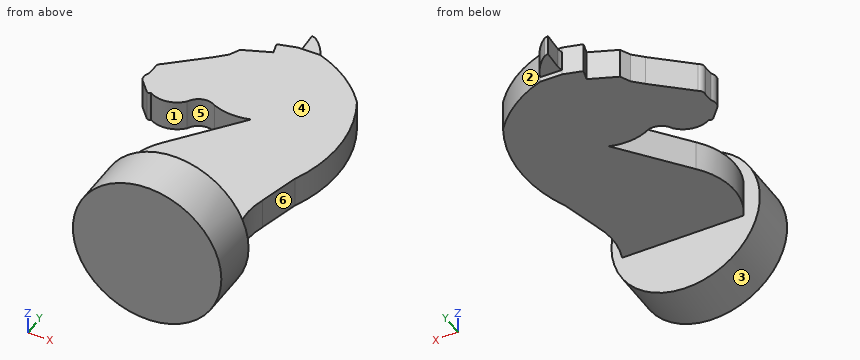
Autodesk Fusion 360 part; units mm, degrees
sketch "Base" plane through (0, 0, 0) normal (0, 0, 1) x (1, 0, 0)
  line L0 (1.35, -11.2) -> (8.7, -11.2)
  line L1 (8.7, -11.2) -> (8.7, -16.1)
  line L2 (8.7, -16.1) -> (1.35, -16.1)
  line L3 (1.35, -16.1) -> (1.35, -11.2)
  line L4 (1.35, -11.2) -> (1.35, -16.5) construction
revolve "Revolve1" add sketch "Base" angle 360 about axis through (1.35, -11.2, 0) along (0, -1, 0)
sketch "Sketch5" plane through (0, 0, 0) normal (0, 0, 1) x (1, 0, 0)
  line L0 (-3.8612, -3.6216) -> (1.2602, 2.7884)
  arc A0 (-2.4491, 2.9542) -> (-4.7968, 2.2709) centre (-3.3362, 1.6273) ccw
  arc A1 (-8.56, 1.8217) -> (-8.1023, 1.7795) centre (-8.3154, 1.9715) ccw
  arc A2 (-8.1023, 1.7795) -> (-4.7968, 2.2709) centre (-6.7484, 4.0355) ccw
  line L1 (-8.4888, 1.7431) -> (-9.6537, 3.0304)
  arc A3 (-9.5649, 4.0683) -> (-9.6537, 3.0304) centre (-8.6269, 3.4652) ccw
  line L2 (-9.5649, 4.0683) -> (-9.5, 4.9)
  arc A4 (-8.7221, 5.7752) -> (-9.5, 4.9) centre (-8.9, 5.15) ccw
  line L3 (-9.1971, 5.7281) -> (-5.657, 8.7735)
  arc A5 (-2.8723, 3.1545) -> (1.2602, 2.7884) centre (-0.3699, 7.8942) ccw
  line L4 (-3.8561, -11.9399) -> (7.9881, -11.9399)
  arc A6 (-3.8612, -3.6216) -> (-3.8561, -11.9399) centre (1.0426, -7.7778) ccw
  line L5 (-5.657, 8.7735) -> (-4.7, 9.7)
  line L6 (-4.7, 9.7) -> (-4.2, 10.7)
  line L7 (-4.2, 10.7) -> (-1.5, 11.8)
  line L8 (-1.5, 11.8) -> (-1.8, 12.9)
  line L9 (-1.8, 12.9) -> (0.0589, 13.407)
  line L10 (0.1583, 14.0219) -> (0.05, 16.1)
  arc A7 (0.0589, 13.407) -> (0.1571, 14.0443) centre (-1.3706, 13.9535) ccw
  arc A8 (2.2064, 13.4396) -> (0.05, 16.1) centre (-2.8988, 11.5057) ccw
  arc A9 (8.1474, 9.2996) -> (2.2064, 13.4396) centre (-1.7746, 1.394) ccw
  line L11 (8.5157, -2.5354) -> (7.2902, -7.2588)
  arc A10 (0.4921, 15.7841) -> (0.0594, 15.92) centre (-3.7578, 3.0059) ccw
  arc A11 (8.5157, -2.5354) -> (8.1474, 9.2996) centre (-3.7578, 3.0059) ccw
  arc A12 (7.4885, -6.4944) -> (7.9881, -11.9399) centre (14.1451, -8.6294) ccw
  line L12 (2.2064, 13.4396) -> (0.0589, 13.407)
extrude "Extrude1" add sketch "Sketch5" along normal mid plane 3 contours L0 A0 A1 A2 L1 A3 L2 A4 L3 A5 L4 A6 L5 L6 L7 L8 L9 A9 L11 A11 A12 L12
extrude "Extrude2" add sketch "Sketch5" along normal mid plane 2 contours L10 A7 A8 A10 L12
Input: part model. Units: mm. Frame: model coordinates. Face numbers are marked on the shaded views. A direction names the side the tool comes from. Round coordinates to 2 decimals unless told otherwise and drop trailing zeros. Loops run counter-clockwise (first coordinate to the right, second up) from the corner with the lowest first, then second, coordinate; pieces in that order, holes last. Notation, with made-up numbers: (81.25, 40.5) -> (98.25, 40.5) arc R21 cw to (98.25, 72.5) -> close; hole circle Ø6 at (4.25, 80.25). An arc over 180 degrees is marked (long way). Answer as a JSON object with one key per item and string values. Group by question number.
1) Draft query along X for the marked faces 1, 2 and 3. Return one class per face: +X half, -X half, draft (parallel to the pull), parting line (faces both ways), or undercut.
2) Pin query (flat end, axial travel): pin 1 (4 mm diameter, centred on y = -5, z = -1, fed in from +X); pin 2 (3 mm diameter, centred on x = -2, z = 1, fed in from +Y); pin 3 (1.1 mm diameter, centred on x = 0.5, y = 15, fed in from +Z). Return the tip coordinate at first contact, or that it passes through.
3) Section query A-A on x = -3.5. Output: boundary loops of the cut face in (y, z) (3 decimals), plus the area to 3 significant figures.
4) Reachability of the marked faces 4, 5 and 6 from +Z, -Z, +X, -X, +Y, -Y: full face, straight path, thin tool, end or side. Return the list, or none.
5) Section query D-D on y = -0.5. Output: boundary loops of the cut face in (x, z).
6) Section query C-C on x = 5.75. Output: boundary loops of the cut face in (y, z), plus the area to 3 significant figures.
7) Ray query, L1, parallel to Z at x = 0.25, y = 8; L2, parallel to Y at x = 1.5, z = 5; L3, parallel to Y at x = -2.75, z = 1. Return the intervals inside material, ascending.
Reply:
{
 "1": {"face 1": "undercut", "face 2": "+X half", "face 3": "parting line"},
 "2": {"pin 1": "stops at x = 8.4", "pin 2": "stops at y = 13.25", "pin 3": "stops at z = 1"},
 "3": {"outline": "(-16.1, -5.523) -> (-11.2, -5.523) -> (-11.2, -1.5) -> (-3.17, -1.5) -> (-3.17, 1.5) -> (-11.2, 1.5) -> (-11.2, 5.523) -> (-16.1, 5.523) -> close; (3.215, -1.5) -> (10.985, -1.5) -> (10.985, 1.5) -> (3.215, 1.5) -> close", "area": "102 mm2"},
 "4": {"face 4": "+Z, +X, -X, +Y", "face 5": "+Z, -Z", "face 6": "+Z, -Z, +X"},
 "5": {"outline": "(-1.37, -1.5) -> (9.24, -1.5) -> (9.24, 1.5) -> (-1.37, 1.5) -> close"},
 "6": {"outline": "(-16.1, -5.89) -> (-11.2, -5.89) -> (-11.2, -1.5) -> (11.61, -1.5) -> (11.61, 1.5) -> (-11.2, 1.5) -> (-11.2, 5.89) -> (-16.1, 5.89) -> close", "area": "126 mm2"},
 "7": {"L1": "z = -1.5 to 1.5", "L2": "y = -16.1 to -11.2", "L3": "y = -16.1 to -2.23, 3.11 to 11.29"}
}
